Job drawing, mm, ordinate dimensions from the low corner. One solid piece. Coordinates: 2 decimals unless noted, no trailing zeros. Write each loop counter-clockwise with the first axis right and the second up, starting at its lowest first coordinate (ties: lowest second). Pieces come first, ordered by that corner, then holes. Notation, with made-up numbers: (54.25, -30) - (69.25, -30) arc R27 ccw to (69.25, 4) - close; hole circle Ø6 at (-26.75, 29). An arc over 180 degrees is marked (long way). Use one line per item in the form item = value. Start each with the question number.
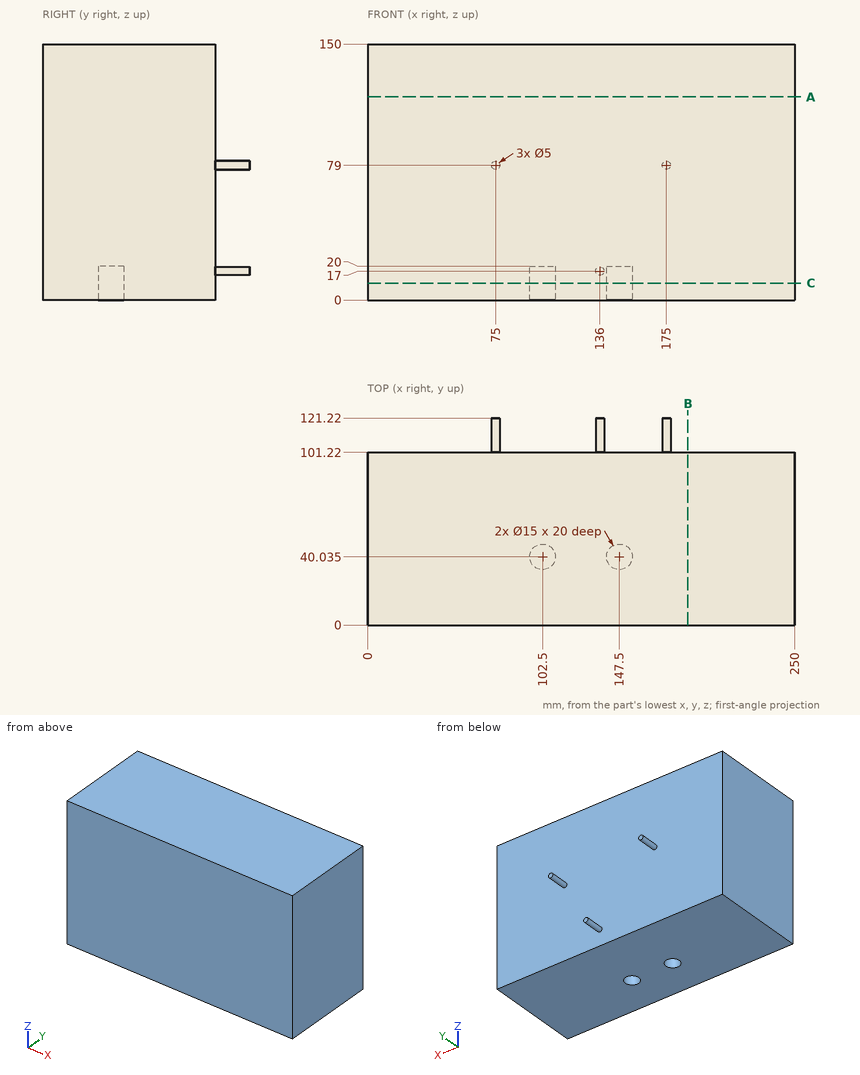
Q1. Drill centre lines: probe 1 along Y at (x, z) = (102.5, 6.5) (3 decimals); probe 2 along Y at (x, z) = (102, 6); probe 3 along Y at (x, z) = (58.5, 103.5). Where is each one in solid material? Low to high.
Q2. Pin check, flat tips, straight feed: P1, Ø4, axis at x = 128.5, z = 91.5, coming from the -Y side; P2, Ø4.5, axis at x = 105.5, y = 43.5, coming from the -Z side; P3, Ø2, axis at x = 50.5, z = 26, coming from the +Y side; P4, Ø6, axis at y = 105.5, z = 53, coming from the +X side. Stop position of each tip, or through.
Q3. Slice it at C-C (z = 10). List the corners of the cut face in (x, y) (3 decimals).
Q4. Slice it at A-A (z = 119). List the corners of the cut face in (x, y), plus the area to 3 significant figures.
Q5. Slice it at B-B (x = 187.5). List the corners of the cut face in (y, z).
Solution:
q1.probe_1 = 0 to 32.535, 47.535 to 101.22
q1.probe_2 = 0 to 32.55, 47.52 to 101.22
q1.probe_3 = 0 to 101.22
q2.P1 = 0
q2.P2 = 20
q2.P3 = 101.22
q2.P4 = through
q3.outline = (0, 0) - (250, 0) - (250, 101.22) - (0, 101.22) - close; hole circle Ø15 at (102.5, 40.035); hole circle Ø15 at (147.5, 40.035)
q4.outline = (0, 0) - (250, 0) - (250, 101.22) - (0, 101.22) - close
q4.area = 25,300 mm2
q5.outline = (0, 0) - (101.22, 0) - (101.22, 150) - (0, 150) - close
